Part model, mm, in its own coordinate system. Coordinates: 2 decimals unless noted, no trailing zeros. Write each loop counter-clockwise with the first axis right and the second up, starting at its lowest first coordinate (ties: lowest second). Pieces come first, ordered by that corner, then holes. Notation, with made-up numbers: (7.25, 39) -> (52.25, 39) arc R25 ccw to (52.25, 72) -> close; hole circle Ø9 at (62.5, -19). An arc over 180 degrees is marked (long way). Write item = value, one per line. Start each with the question number.
Q1. Band-saw the part on B-B, the plane x = 22. List the corners of the cut face in (y, z), plus the area to 3 significant figures.
Q2. Band-saw the part on C-C, the plane y = -36.5. List the corners of the cut face in (x, z).
Q3. Pin check, flat tips, straight feed: P1, Ø1, axis at y = -143.5, z = 1.5, coming from the +X side; P2, Ø1.6, axis at y = 2, z = 2, coming from the -X side. Stop position of each tip, or through.
Q4. Band-saw the part on D-D, the plane z = 2.65. Give the number of separate pieces and of enclosed holes in the cut face, plus the area to 3 significant figures.
Q5. Band-saw the part on A-A, the plane x = -35.5. List the corners of the cut face in (y, z), plus the area to 3 significant figures.
Q6. Probe line 1 (Y direction, x = 63.5, z = 2); line 2 (Y direction, x = 61, z = 2.65); line 3 (X direction, y = 25.5, z = 3.35). List the from-to ranges inside material, lowest first.
from build123d import *

# Parameters (mm, degrees)
SKETCH1_W           = 151
SKETCH1_H           = 253
BOSS_EXTRUDE1_DEPTH = 4
SKETCH2_W           = 52.50306414
SKETCH2_H           = 122.00289527
CUT_EXTRUDE1_DEPTH  = 5
CUT_EXTRUDE4_DEPTH  = 5
SKETCH8_R           = 2
CUT_EXTRUDE6_DEPTH  = 5
SKETCH10_R          = 4
SKETCH10_R_2        = 2
BOSS_EXTRUDE3_DEPTH = 4
SKETCH11_W          = 24.2
SKETCH11_H          = 30.2
CUT_EXTRUDE9_DEPTH  = 10
SKETCH16_W          = 118.99693586
SKETCH16_H          = 82
BOSS_EXTRUDE4_DEPTH = 4
BOSS_EXTRUDE5_DEPTH = 4
CUT_EXTRUDE13_DEPTH = 10
SKETCH27_W          = 20
SKETCH27_H          = 53
CUT_EXTRUDE14_DEPTH = 5
SKETCH29_W          = 20.5
SKETCH29_H          = 4
BOSS_EXTRUDE6_DEPTH = 4
SKETCH31_W          = 30
SKETCH31_H          = 5
SKETCH31_W_2        = 15.03868673
SKETCH31_W_3        = 20
SKETCH31_H_2        = 4
CUT_EXTRUDE16_DEPTH = 10
SKETCH32_R          = 2
CUT_EXTRUDE17_DEPTH = 10


with BuildPart() as part:
    # Sketch1 → Boss-Extrude1 (new body)
    with BuildSketch(Plane.XY):
        with Locations((0, -1)):
            Rectangle(SKETCH1_W, SKETCH1_H)
    extrude(amount=BOSS_EXTRUDE1_DEPTH)

    # Sketch2 → Cut-Extrude1 (cut)
    with BuildSketch(Plane.XY.offset(4)):
        with Locations((-49.24846793, -66.498552365)):
            Rectangle(SKETCH2_W, SKETCH2_H)
    extrude(amount=-CUT_EXTRUDE1_DEPTH, mode=Mode.SUBTRACT)

    # Sketch5 → Cut-Extrude4 (cut)
    with BuildSketch(Plane.XY.offset(4)):
        with BuildLine():
            Line((-61.5, 0.50289527), (-61.5, 2.50289527))
            ThreePointArc((-61.5, 2.50289527), (-60.5, 3.50289527), (-59.5, 2.50289527))
            Line((-59.5, 2.50289527), (-59.5, 0.50289527))
            ThreePointArc((-59.5, 0.50289527), (-60.5, -0.49710473), (-61.5, 0.50289527))
        make_face()
        with BuildLine():
            Line((-56.5, 0.50289527), (-56.5, 2.50289527))
            ThreePointArc((-56.5, 2.50289527), (-55.5, 3.50289527), (-54.5, 2.50289527))
            Line((-54.5, 2.50289527), (-54.5, 0.50289527))
            ThreePointArc((-54.5, 0.50289527), (-55.5, -0.49710473), (-56.5, 0.50289527))
        make_face()
    extrude(amount=-CUT_EXTRUDE4_DEPTH, mode=Mode.SUBTRACT)

    # Sketch8 → Cut-Extrude6 (cut)
    with BuildSketch(Plane.XY.offset(4)):
        with Locations((-73, 79.562158061)):
            Circle(SKETCH8_R)
    extrude(amount=-CUT_EXTRUDE6_DEPTH, mode=Mode.SUBTRACT)

    # Sketch10 → Boss-Extrude3 (add)
    with BuildSketch(Plane.XY.offset(4)):
        with Locations((-73, 79.562158061)):
            Circle(SKETCH10_R)
        with Locations((-73, 79.562158061)):
            Circle(SKETCH10_R_2, mode=Mode.SUBTRACT)
    extrude(amount=-BOSS_EXTRUDE3_DEPTH)

    # Sketch11 → Cut-Extrude9 (cut)
    with BuildSketch(Plane(origin=(0, 0, 0), x_dir=(-1, 0, 0), z_dir=(0, 0, -1))):
        with Locations((58.4, 26.6)):
            Rectangle(SKETCH11_W, SKETCH11_H)
    extrude(amount=-CUT_EXTRUDE9_DEPTH, mode=Mode.SUBTRACT)

    # Sketch16 → Boss-Extrude4 (add)
    with BuildSketch(Plane.XY.offset(4)):
        with Locations((16.00153207, -168.5)):
            Rectangle(SKETCH16_W, SKETCH16_H)
    extrude(amount=-BOSS_EXTRUDE4_DEPTH)

    # Sketch24 → Boss-Extrude5 (add)
    with BuildSketch(Plane.XY.offset(4)):
        with BuildLine():
            Line((-43.49693586, -209.5), (-43.49693586, -140.130236158))
            add(Edge.make_bspline(
                [(-73.5, -209.5), (-66.548744275, -187.160783495), (-43.937613379, -164.067684131), (-43.49693586, -140.130236158)],
                knots=[0, 0, 0, 0, 0.851213122, 0.851213122, 0.851213122, 0.851213122], degree=3))
            Line((-73.5, -209.5), (-43.49693586, -209.5))
        make_face()
    extrude(amount=-BOSS_EXTRUDE5_DEPTH)

    # Sketch26 → Cut-Extrude13 (cut)
    with BuildSketch(Plane.XY.offset(4)):
        with BuildLine():
            Line((-44, -178.3), (-44, -209.5))
            Line((-44, -209.5), (41, -209.5))
            Line((41, -209.5), (41, -178.3))
            ThreePointArc((41, -178.3), (-1.5, -135.8), (-44, -178.3))
        make_face()
    extrude(amount=-CUT_EXTRUDE13_DEPTH, mode=Mode.SUBTRACT)

    # Sketch27 → Cut-Extrude14 (cut)
    with BuildSketch(Plane.XY.offset(4)):
        with Locations((65.5, -154)):
            Rectangle(SKETCH27_W, SKETCH27_H)
    extrude(amount=-CUT_EXTRUDE14_DEPTH, mode=Mode.SUBTRACT)

    # Sketch29 → Boss-Extrude6 (add)
    with BuildSketch(Plane.XY.offset(4)):
        with Locations((-33.24693586, -125.5)):
            Rectangle(SKETCH29_W, SKETCH29_H)
    extrude(amount=-BOSS_EXTRUDE6_DEPTH)

    # Sketch31 → Cut-Extrude16 (cut)
    with BuildSketch(Plane.XY.offset(4)):
        with Locations((40.5, 123)):
            Rectangle(SKETCH31_W, SKETCH31_H)
        with Locations((-40.5, 123)):
            Rectangle(SKETCH31_W, SKETCH31_H)
        with Locations((60.155656635, 47)):
            Rectangle(SKETCH31_W_2, SKETCH31_H)
        with Locations((30.5, -10)):
            Rectangle(SKETCH31_W, SKETCH31_H)
        with Locations((6.5, -60)):
            Rectangle(SKETCH31_W_3, SKETCH31_H)
        with Locations((-54.75, 47)):
            Rectangle(SKETCH31_W_3, SKETCH31_H)
        with Locations((24.5, -125.5)):
            Rectangle(SKETCH31_W, SKETCH31_H_2)
    extrude(amount=-CUT_EXTRUDE16_DEPTH, mode=Mode.SUBTRACT)

    # Sketch32 → Cut-Extrude17 (cut)
    with BuildSketch(Plane.XY.offset(4)):
        with Locations((60.936739195, -10)):
            Circle(SKETCH32_R)
    extrude(amount=-CUT_EXTRUDE17_DEPTH, mode=Mode.SUBTRACT)


solid = part.part
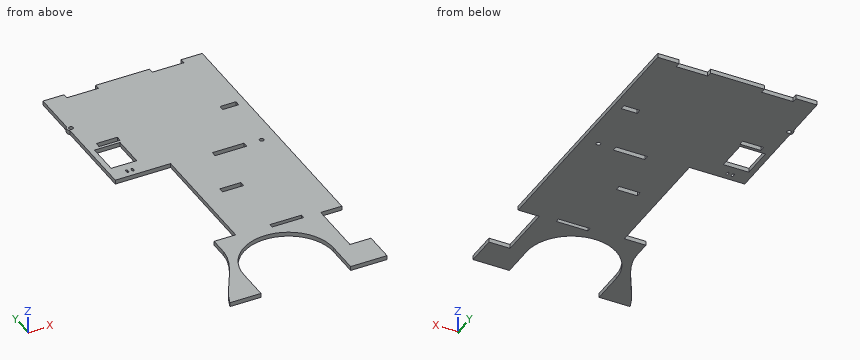
Ans:
q1.outline = (-142.89, 0) -> (-127.5, 0) -> (-127.5, 4) -> (-142.89, 4) -> close; (-123.5, 0) -> (-12.5, 0) -> (-12.5, 4) -> (-123.5, 4) -> close; (-7.5, 0) -> (125.5, 0) -> (125.5, 4) -> (-7.5, 4) -> close
q1.area = 1,040 mm2
q2.outline = (-23, 0) -> (75.5, 0) -> (75.5, 4) -> (-23, 4) -> close
q3.P1 = 55.5
q3.P2 = -75.5
q4.separate_pieces = 1
q4.enclosed_holes = 10
q4.area = 34,400 mm2
q5.outline = (-152.8, 0) -> (-123.5, 0) -> (-123.5, 4) -> (-152.8, 4) -> close; (-5.5, 0) -> (120.5, 0) -> (120.5, 4) -> (-5.5, 4) -> close
q5.area = 621 mm2
q6.line_1 = -209.5 to -180.5, -127.5 to 44.5, 49.5 to 125.5
q6.line_2 = -209.5 to -180.5, -127.5 to -12, -8 to 44.5, 49.5 to 125.5
q6.line_3 = -75.5 to -70.5, -46.3 to 75.5
